Geometry: final body of the model. Coordinates: model frame, mm. A direction names the side the tool comes from. Give positions to 0.01 mm unless a question says otherwise; leave off trailing zeros. Order: outer loops, then holes, each group sorted by start corner. A loop starts at its lowest first (then second) coordinate and runs counter-clockwise, first axis right, second up. Notation, with made-up numbers: M 74,51 L 121,51 A11 ccw 121,61 Z; hole C -24,13 d11. An arc over 180 degrees is marked long. Use CSV: the item, a comma, the result in double quotes.
```python
from build123d import *

# Parameters (mm, degrees)
BOSS_EXTRUDE1_DEPTH = 1
SKETCH3_R           = 3.25
CUT_EXTRUDE2_DEPTH  = 10
SKETCH4_R           = 0.75
CUT_EXTRUDE3_DEPTH  = 10


with BuildPart() as part:
    # Sketch1 → Boss-Extrude1 (new body)
    with BuildSketch(Plane.XY):
        with BuildLine():
            Line((-17.017879978, -7), (6.982120022, -7))
            Line((6.982120022, -7), (6.982120022, -5.5))
            Line((6.982120022, -5.5), (6.982120022, -4.5))
            Line((6.982120022, -4.5), (7.982120022, -4.5))
            Line((7.982120022, -4.5), (8.482120022, -4.5))
            ThreePointArc((8.482120022, -4.5), (9.189226803, -4.207106781), (9.482120022, -3.5))
            Line((9.482120022, -3.5), (9.482120022, -0.5))
            ThreePointArc((9.482120022, -0.5), (9.189226803, 0.207106781), (8.482120022, 0.5))
            Line((8.482120022, 0.5), (7.858116823, 0.5))
            ThreePointArc((7.858116823, 0.5), (7.220739384, 0.72944825), (6.87585222, 1.3125))
            ThreePointArc((6.87585222, 1.3125), (1.68605895, 6.793909421), (-5.464373249, 4.375))
            ThreePointArc((-5.464373249, 4.375), (-5.811985297, 4.098612181), (-6.244997998, 4))
            Line((-6.244997998, 4), (-14.017879978, 4))
            ThreePointArc((-14.017879978, 4), (-16.139200322, 3.121320344), (-17.017879978, 1))
            Line((-17.017879978, 1), (-17.017879978, -7))
        make_face()
    extrude(amount=BOSS_EXTRUDE1_DEPTH)

    # Sketch3 → Cut-Extrude2 (cut)
    with BuildSketch(Plane.XY.offset(1)):
        with BuildLine():
            Line((-9.737921814, -0.759288793), (-17.017879978, -4))
            Line((-17.017879978, -4), (-17.017879978, -7))
            Line((-17.017879978, -7), (-9.017879978, -7))
            Line((-9.017879978, -7), (-7.306383876, -6.244499443))
            ThreePointArc((-7.306383876, -6.244499443), (-5.775271325, -2.284229555), (-9.737921814, -0.759288793))
        make_face()
        with BuildLine():
            ThreePointArc((-8.131842017, 2.458113883), (-7.94985551, 2.705621093), (-7.657500368, 2.8))
            Line((-7.657500368, 2.8), (-7.211592921, 2.8))
            ThreePointArc((-7.211592921, 2.8), (-6.805971829, 2.592355142), (-6.737251272, 2.141886117))
            Line((-6.737251272, 2.141886117), (-7.403917939, 0.141886117))
            ThreePointArc((-7.403917939, 0.141886117), (-7.585904446, -0.105621093), (-7.878259588, -0.2))
            Line((-7.878259588, -0.2), (-8.324167035, -0.2))
            ThreePointArc((-8.324167035, -0.2), (-8.729788127, 0.007644858), (-8.798508684, 0.458113883))
            Line((-8.798508684, 0.458113883), (-8.131842017, 2.458113883))
        make_face()
        with BuildLine():
            ThreePointArc((-5.298508684, 0.341886117), (-5.229788127, 0.792355142), (-4.824167035, 1))
            Line((-4.824167035, 1), (-4.378259588, 1))
            ThreePointArc((-4.378259588, 1), (-4.085904446, 0.905621093), (-3.903917939, 0.658113883))
            Line((-3.903917939, 0.658113883), (-3.237251272, -1.341886117))
            ThreePointArc((-3.237251272, -1.341886117), (-3.305971829, -1.792355142), (-3.711592921, -2))
            Line((-3.711592921, -2), (-4.157500368, -2))
            ThreePointArc((-4.157500368, -2), (-4.44985551, -1.905621093), (-4.631842017, -1.658113883))
            Line((-4.631842017, -1.658113883), (-5.298508684, 0.341886117))
        make_face()
        Circle(SKETCH3_R)
    extrude(amount=-CUT_EXTRUDE2_DEPTH, mode=Mode.SUBTRACT)

    # Sketch4 → Cut-Extrude3 (cut)
    with BuildSketch(Plane.XY.offset(1)):
        with Locations((-14.517879978, 3)):
            Circle(SKETCH4_R)
        with Locations((-16.017879978, -1.5)):
            Circle(SKETCH4_R)
        with Locations((7.782120022, -0.7)):
            Circle(SKETCH4_R)
        with Locations((6.732120022, -3.7)):
            Circle(SKETCH4_R)
    extrude(amount=-CUT_EXTRUDE3_DEPTH, mode=Mode.SUBTRACT)


solid = part.part
```
1. Pin query (flat end, axial travel): pin 1 Ø0.5 at (y, z) = (-5.5, 0.5) entering from +X. Return the tip coordinate at first contact, or that it passes through.
Answer:
pin 1,"x = 6.98"
2. Pull-direction query (X, two-part tool) for faces 4 (the face through (7.23, 0.72, 0.49)), 5 (the face through (-7.066, 1.156, 0.507)), 6 (the face through (7.7, -4.5, 0.5)); classes: +X half, -X half, draft (parallel to the pull), parting line (faces both ways), or undercut.
Answer:
face 4,"+X half"
face 5,"undercut"
face 6,"draft"
3. Section B-B, the plane y = 3.5. Return the cut outline in (x, z).
Answer:
outline,"M -15.68,0 L -15.08,0 L -15.08,1 L -15.68,1 Z; M -13.96,0 L 6.06,0 L 6.06,1 L -13.96,1 Z"
4. Line query: line 1 (Y direction, x = 7.25, z = 0.75); line 2 (X direction, y = -1, z = 0.2); line 3 (X direction, y = -1.75, z = 0.15). Output: solid intervals per line, ascending.
Answer:
line 1,"-4.5 to -4.24, -3.16 to -1.23, -0.17 to 0.71"
line 2,"-17.02 to -16.58, -15.46 to -10.28, -6.86 to -4.85, -3.35 to -3.09, 3.09 to 7.09, 8.47 to 9.48"
line 3,"-17.02 to -16.72, -15.31 to -11.96, -6.08 to -4.59, -3.28 to -2.74, 2.74 to 9.48"
5. Reachability of faces 1 (the face through (-4.96, -0.67, 0.51)), 2 (the face through (6.982, -5.8, 0.5)), 3 (the face through (9.482, -2, 0.5)) from +Z, -Z, +X, -X, +Y, -Y: full face, straight path, thin tool, end or side. Return the list, or none.
Answer:
face 1,"+Z, -Z"
face 2,"+Z, -Z, +X, -Y"
face 3,"+Z, -Z, +X, +Y, -Y"
6. Section C-C, the plane z = 0.15. Give the number of separate pieces and of enclosed holes in the cut face, plus the area to 3 significant figures.
Answer:
separate pieces,"1"
enclosed holes,"7"
area,"193 mm2"
7. Section A-A, the plane x = 0. Return the cut outline in (y, z).
Answer:
outline,"M -7,0 L -3.25,0 L -3.25,1 L -7,1 Z; M 3.25,0 L 7,0 L 7,1 L 3.25,1 Z"
